Design review of the part built by this model. Coordinates are the model's own, in mm. Face numbers are marked on the shaded views. A direction names the side the tool comes from. Give positions to 0.01 mm unless a question says otherwise; leave off trailing zeros. Write each loop counter-clockwise with the first axis right and the second up, starting at its lowest first coordinate (ties: lowest second). Pieces come first, ordered by that corner, then holes. Notation, with made-up numbers: M 5.5,-12 L 28.5,-12 A23 cw 28.5,16 Z; hole C -11,28 d4. An arc over 180 degrees is marked long. Use one line per item in the form item = value. Start each with the question number.
from build123d import *

# Parameters (mm, degrees)
CYLINDER108_R          = 1.8
CYLINDER108_DEPTH      = 10
CYLINDER111_R          = 1.8
CYLINDER111_DEPTH      = 10
CYLINDER109_R          = 1.8
CYLINDER109_DEPTH      = 10
CYLINDER110_R          = 1.8
CYLINDER110_DEPTH      = 10
CYLINDER106_R          = 2.5
CYLINDER106_DEPTH      = 24
CYLINDER107_R          = 11.3
CYLINDER107_DEPTH      = 6
BOX038_W               = 42.3
BOX038_H               = 39.8
BOX038_DEPTH           = 42.3
CYLINDER102_R          = 6.2
CYLINDER102_DEPTH      = 30
CYLINDER103_R          = 2.1
CYLINDER103_DEPTH      = 10
CYLINDER104_R          = 6.2
CYLINDER104_DEPTH      = 30
CYLINDER105_R          = 2.1
CYLINDER105_DEPTH      = 10
BOX037_W               = 47
BOX037_H               = 4
BOX037_DEPTH           = 50
BOX036_W               = 43
BOX036_H               = 40
BOX036_DEPTH           = 11
EXTRUDE_DEPTH          = 4
CUT097_PLACEMENT_ANGLE = 180


with BuildPart() as cylinder108:
    # Cylinder108 → Cylinder108 (new body)
    with BuildSketch(Plane(origin=(5.65, 0, 36.65), x_dir=(1, 0, 0), z_dir=(0, -1, 0))):
        Circle(CYLINDER108_R)
    extrude(amount=CYLINDER108_DEPTH)


with BuildPart() as cylinder111:
    # Cylinder111 → Cylinder111 (new body)
    with BuildSketch(Plane(origin=(36.65, 0, 36.65), x_dir=(1, 0, 0), z_dir=(0, -1, 0))):
        Circle(CYLINDER111_R)
    extrude(amount=CYLINDER111_DEPTH)


with BuildPart() as cylinder109:
    # Cylinder109 → Cylinder109 (new body)
    with BuildSketch(Plane(origin=(5.65, 0, 5.65), x_dir=(1, 0, 0), z_dir=(0, -1, 0))):
        Circle(CYLINDER109_R)
    extrude(amount=CYLINDER109_DEPTH)


with BuildPart() as cylinder110:
    # Cylinder110 → Cylinder110 (new body)
    with BuildSketch(Plane(origin=(36.65, 0, 5.65), x_dir=(1, 0, 0), z_dir=(0, -1, 0))):
        Circle(CYLINDER110_R)
    extrude(amount=CYLINDER110_DEPTH)


with BuildPart() as cylinder106:
    # Cylinder106 → Cylinder106 (new body)
    with BuildSketch(Plane(origin=(21.15, -2, 21.15), x_dir=(1, 0, 0), z_dir=(0, -1, 0))):
        Circle(CYLINDER106_R)
    extrude(amount=CYLINDER106_DEPTH)


with BuildPart() as cylinder107:
    # Cylinder107 → Cylinder107 (new body)
    with BuildSketch(Plane(origin=(21.15, 0, 21.15), x_dir=(1, 0, 0), z_dir=(0, -1, 0))):
        Circle(CYLINDER107_R)
    extrude(amount=CYLINDER107_DEPTH)


with BuildPart() as fusion050:
    # Box038 → Box038 (new body)
    with BuildSketch(Plane.XY):
        with Locations((21.15, 19.9)):
            Rectangle(BOX038_W, BOX038_H)
    extrude(amount=BOX038_DEPTH)

    # Fusion048: union Cylinder107
    add(cylinder107.part)

    # Fusion049: union Cylinder106
    add(cylinder106.part)

    # Fusion050: union Cylinder108, Cylinder111, Cylinder109, Cylinder110
    add(cylinder108.part)
    add(cylinder111.part)
    add(cylinder109.part)
    add(cylinder110.part)


with BuildPart() as fusion050_1:
    # Fusion050 placement: moved
    add(fusion050.part.moved(Location((9, 0, 11))))


with BuildPart() as cylinder102:
    # Cylinder102 → Cylinder102 (new body)
    with BuildSketch(Plane.XY.offset(10)):
        Circle(CYLINDER102_R)
    extrude(amount=CYLINDER102_DEPTH)


with BuildPart() as fusion046:
    # Cylinder103 → Cylinder103 (new body)
    with BuildSketch(Plane.XY):
        Circle(CYLINDER103_R)
    extrude(amount=CYLINDER103_DEPTH)

    # Fusion046: union Cylinder102
    add(cylinder102.part)


with BuildPart() as fusion046_1:
    # Fusion046 placement: moved
    add(fusion046.part.moved(Location((22, 12, -5))))


with BuildPart() as cylinder104:
    # Cylinder104 → Cylinder104 (new body)
    with BuildSketch(Plane.XY.offset(10)):
        Circle(CYLINDER104_R)
    extrude(amount=CYLINDER104_DEPTH)


with BuildPart() as fusion047:
    # Cylinder105 → Cylinder105 (new body)
    with BuildSketch(Plane.XY):
        Circle(CYLINDER105_R)
    extrude(amount=CYLINDER105_DEPTH)

    # Fusion047: union Cylinder104
    add(cylinder104.part)


with BuildPart() as fusion047_1:
    # Fusion047 placement: moved
    add(fusion047.part.moved(Location((41, 29, -5))))


with BuildPart() as box037:
    # Box037 → Box037 (new body)
    with BuildSketch(Plane(origin=(52, 0, 0), x_dir=(-1, 0, 0), z_dir=(0, 0, 1))):
        with Locations((23.5, 2)):
            Rectangle(BOX037_W, BOX037_H)
    extrude(amount=BOX037_DEPTH)


with BuildPart() as box036:
    # Box036 → Box036 (new body)
    with BuildSketch(Plane(origin=(9, 0, 0), x_dir=(1, 0, 0), z_dir=(0, 0, 1))):
        with Locations((21.5, 20)):
            Rectangle(BOX036_W, BOX036_H)
    extrude(amount=BOX036_DEPTH)


with BuildPart() as obj1:
    # Sketch024 → Extrude (new body)
    with BuildSketch(Plane.YZ):
        Polygon((0, 0), (0, 50), (22, 50), (40, 11), (40, 0), align=None)
    extrude(amount=-EXTRUDE_DEPTH)


with BuildPart() as obj1_1:
    # Extrude placement: moved
    add(obj1.part.moved(Location((9, 0, 0))))

    # Fusion045: union Box037, Box036
    add(box037.part)
    add(box036.part)

    # Cut095: cut Fusion047
    add(fusion047_1.part, mode=Mode.SUBTRACT)

    # Cut096: cut Fusion046
    add(fusion046_1.part, mode=Mode.SUBTRACT)

    # Cut097: cut Fusion050
    add(fusion050_1.part, mode=Mode.SUBTRACT)


with BuildPart() as obj1_2:
    # Cut097 placement: moved
    add(obj1_1.part.moved(Location((57, 6.5, 0))).rotate(Axis((57, 6.5, 0), (0, 0, 1)), CUT097_PLACEMENT_ANGLE))


solid = obj1_2.part
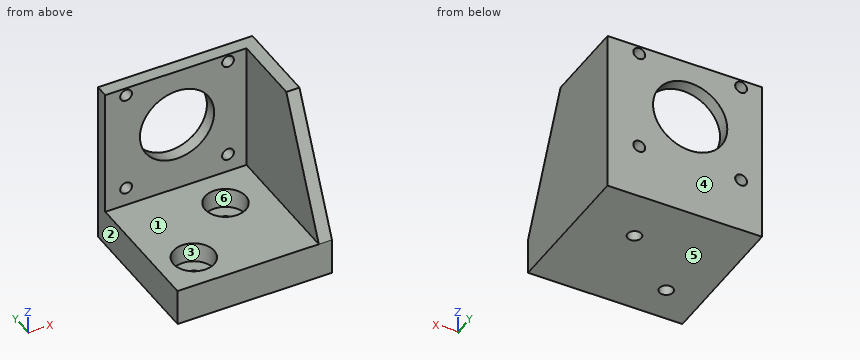
1. Clearance check with flat-ended pins moving along their axes: pin 1 Ø1.5 at (y, z) = (-0.5, 20.5) entering from -X; pin 2 Ø3 at (x, z) = (11.35, 16.65) entering from -Y; pin 3 Ø6.5 at (x, y) = (35, -5.5) entering from +Z; pin 4 Ø1 at (x, y) = (42.5, -23) entering from +Z. State where each tip first meets the part, or that it passes through.
2. We need section B-B (z = 47.65). State the section outline as (x, y) points.
3. For the marked faces 1 and 2, list the 3-axis set-ups (+Z, -Z, +X, -X, +Y, -Y) from which the entire face can be reached by the end or side of a thin tool; tool diameter is ignored.
4. We need section A-A (y = -5.5). State the section outline as (x, z) points.
5. We need section D-D (z = 29). State the section outline as (x, y) points, and give its area (3 significant figures).
6. To check wall thickness, follow L1, parallel to X at y = 9, z = 16.65; L2, parallel to Z at x = 11.35, y = 8.85; L3, parallel to Y at x = 16, z = 9.55. State the ranges of each line that lie inside material, in increasing order.
7. Draft analysis for pull direction Y (two halves, no side actions). For the marked faces 3, 4, 5 and 6, state which applies: pulls with the +Y half, pulls with the -Y half, needs draft (parallel to the pull), parting line crosses it, or undercut.
8. We need section C-C (z = 7.5). State the section outline as (x, y) points, and give its area (3 significant figures).
Answer block:
q1.pin_1 = 48
q1.pin_2 = through
q1.pin_3 = 5
q1.pin_4 = 11
q2.outline = M 5,6.5 L 9.55,6.5 L 9.55,10.5 L 5,10.5 Z; M 13.15,6.5 L 40.55,6.5 L 40.55,10.5 L 13.15,10.5 Z; M 44.15,6.5 L 48,6.5 L 48,-16.58 L 52,-16.58 L 52,10.5 L 44.15,10.5 Z
q3.face_1 = +Z, -X, -Y
q3.face_2 = +Z, -Z, -X, +Y, -Y
q4.outline = M 5,0 L 32.9,0 L 32.9,5 L 28.8,5 L 28.8,11 L 5,11 Z; M 37.1,0 L 52,0 L 52,50 L 48,50 L 48,11 L 41.2,11 L 41.2,5 L 37.1,5 Z
q5.outline = M 5,6.5 L 16,6.5 L 16,10.5 L 5,10.5 Z; M 37.7,6.5 L 48,6.5 L 48,-25.19 L 52,-25.19 L 52,10.5 L 37.7,10.5 Z
q5.area = 228 mm^2
q6.L1 = 5 to 9.55, 13.15 to 40.55, 44.15 to 52
q6.L2 = 0 to 14.85, 18.45 to 45.85, 49.45 to 50
q6.L3 = -33.5 to -28.7, -16.3 to 10.5
q7.face_3 = undercut
q7.face_4 = pulls with the +Y half
q7.face_5 = needs draft
q7.face_6 = undercut
q8.outline = M 5,-33.5 L 52,-33.5 L 52,10.5 L 5,10.5 Z; hole C 16,-22.5 d12.4; hole C 35,-5.5 d12.4
q8.area = 1,830 mm^2
